For this review, use the dimensioned drawing (mm, ordinates from the lowest corner) and the shaded views. Round coordinates to 2 decimals unless told otherwise and drop trailing zeros. Order: outer loops, then holes, each group sorted by start corner. A loop starts at its lowest first (then second) coordinate and runs counter-clockwise, first axis right, second up. Notation, with made-up numbers: (0, -17) -> (40, -17) arc R13 ccw to (40, -6) -> close; hole circle Ø2 at (-30, 41.5). An arc over 180 degrees is marked (long way). Answer in a Markdown table with one row per item.
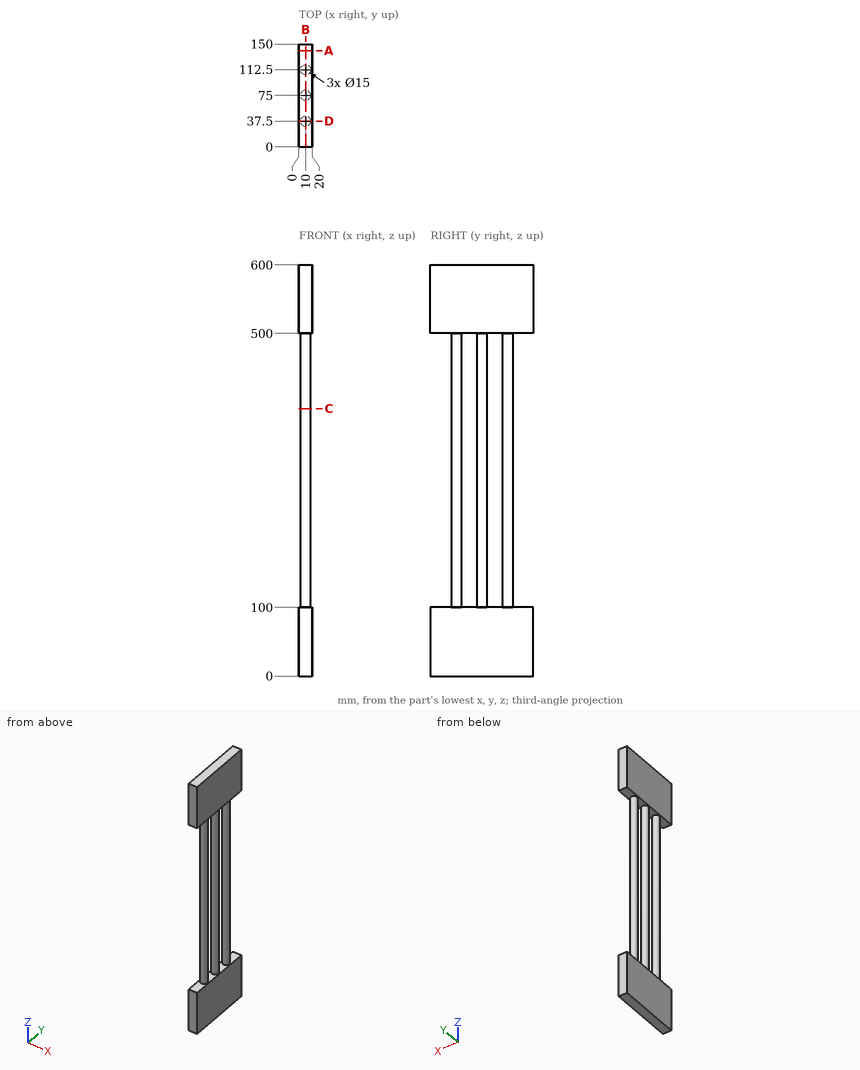
Q1. To check wall thickness, follow probe 1 along Y at (x, z) = (9, 237.5); probe 2 along Z at (x, y) = (10.25, 60.5); probe 3 along Y at (x, z) = (5, 439). State the ranges of each line that lie inside material, in increasing order.
Answer key:
| item | result |
|---|---|
| probe 1 | y = 30.07 to 44.93, 67.57 to 82.43, 105.07 to 119.93 |
| probe 2 | z = 0 to 100, 500 to 600 |
| probe 3 | y = 31.91 to 43.09, 69.41 to 80.59, 106.91 to 118.09 |
Q2. Take a section at D-D, the plane y = 37.5. Write out the cut boundary in (x, z), then the cut area to 3 significant figures.
Answer key:
| item | result |
|---|---|
| outline | (0, 0) -> (20, 0) -> (20, 100) -> (17.5, 100) -> (17.5, 500) -> (20, 500) -> (20, 600) -> (0, 600) -> (0, 500) -> (2.5, 500) -> (2.5, 100) -> (0, 100) -> close |
| area | 10,000 mm^2 |
Q3. Take a section at B-B, the plane x = 10. Write out the cut boundary in (y, z), then the cut area to 3 significant figures.
Answer key:
| item | result |
|---|---|
| outline | (0, 0) -> (150, 0) -> (150, 100) -> (120, 100) -> (120, 500) -> (150, 500) -> (150, 600) -> (0, 600) -> (0, 500) -> (30, 500) -> (30, 100) -> (0, 100) -> close; hole (45, 100) -> (67.5, 100) -> (67.5, 500) -> (45, 500) -> close; hole (82.5, 100) -> (105, 100) -> (105, 500) -> (82.5, 500) -> close |
| area | 48,000 mm^2 |
Q4. Clearance check with flat-ended pins moving along their axes: pin 1 Ø12 at (x, y) = (8, 56) entering from -Z; pin 2 Ø8 at (x, z) = (4, 411.5) entering from -Y; pin 3 Ø1 at (y, z) = (32, 180.5) entering from +X; pin 4 Ø8 at (x, z) = (11, 436.5) entering from +Y. State where each tip first meets the part, or that it passes through.
Answer key:
| item | result |
|---|---|
| pin 1 | stops at z = 0 |
| pin 2 | stops at y = 30.27 |
| pin 3 | stops at x = 15.59 |
| pin 4 | stops at y = 120 |
Q5. Take a section at C-C, the plane z = 390. Write out the cut boundary in (x, y).
Answer key:
| item | result |
|---|---|
| outline | circle Ø15 at (10, 37.5); circle Ø15 at (10, 75); circle Ø15 at (10, 112.5) |
Q6. Take a section at A-A, the plane y = 140.5. Write out the cut boundary in (x, z), then the cut area to 3 significant figures.
Answer key:
| item | result |
|---|---|
| outline | (0, 0) -> (20, 0) -> (20, 100) -> (0, 100) -> close; (0, 500) -> (20, 500) -> (20, 600) -> (0, 600) -> close |
| area | 4,000 mm^2 |
